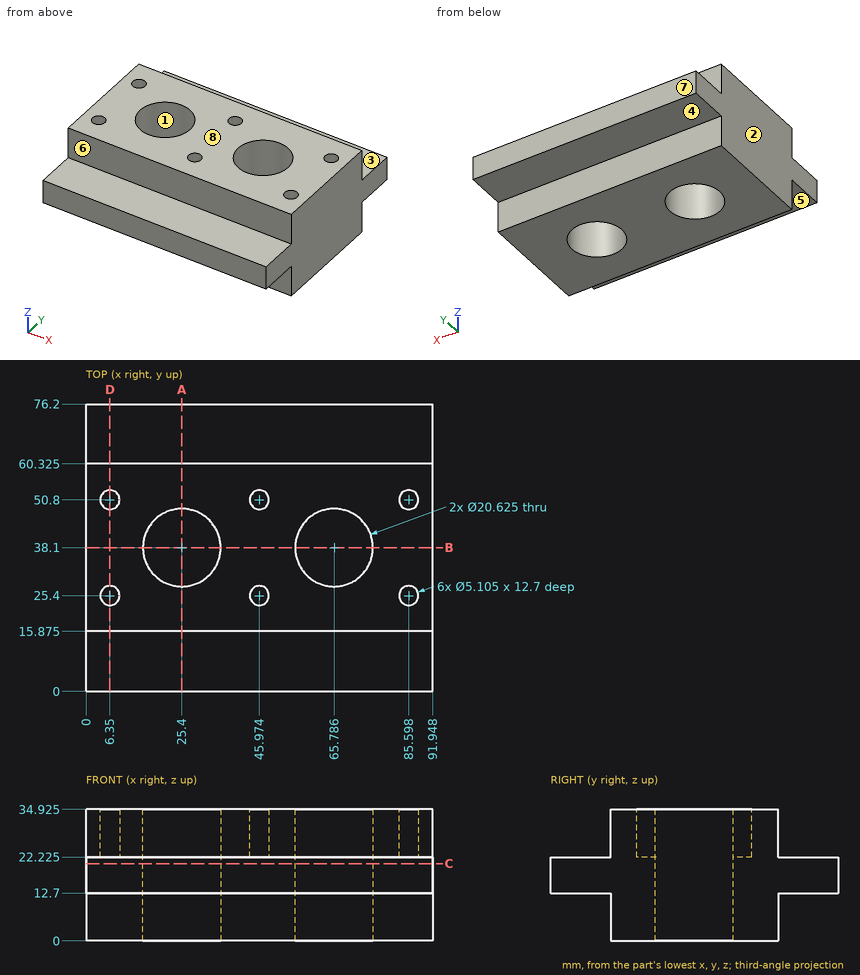
Input: dimensioned drawing with shaded views. Units: mm. Origin: part minimum x, y, z. A direction names the side the tool comes from. Give positions to 0.01 mm unless a question says otherwise; leave off trailing zeros. Order: outer loops, then holes, each group sorted by start corner. A loop starts at its lowest first (then second) coordinate and runs counter-clockwise, first axis right, second up. Notation, with made-up numbers: (-5.5, -9) -> (17.5, -9) arc R12 ccw to (17.5, 5) -> close; hole circle Ø6 at (68.5, 32.5). An arc over 180 degrees is marked (long way). Use a Markdown table: item, result.
1) Ray query, line 1 along X through (y, z) = (44, 12) (1 decimal); line 2 along X through (y, z) = (34, 24) (1 decimal); line 3 along Z through (x, y) = (24, 65.5) (1 decimal). Return the intervals inside material, ascending. Write a range as [from, to].
Answer list:
| item | result |
|---|---|
| line 1 | [0, 16.9], [33.9, 57.3], [74.2, 91.9] |
| line 2 | [0, 15.9], [34.9, 56.3], [75.2, 91.9] |
| line 3 | [12.7, 22.2] |
2) Section query D-D, the plane x = 6.35. Return the cut outline in (y, z) (1 decimal).
Answer list:
| item | result |
|---|---|
| outline | (0, 12.7) -> (15.9, 12.7) -> (15.9, 0) -> (60.3, 0) -> (60.3, 12.7) -> (76.2, 12.7) -> (76.2, 22.2) -> (60.3, 22.2) -> (60.3, 34.9) -> (53.4, 34.9) -> (53.4, 22.2) -> (48.2, 22.2) -> (48.2, 34.9) -> (28, 34.9) -> (28, 22.2) -> (22.8, 22.2) -> (22.8, 34.9) -> (15.9, 34.9) -> (15.9, 22.2) -> (0, 22.2) -> close |
3) Section query B-B, the plane y = 38.1. Return the cut outline in (x, z) (1 decimal).
Answer list:
| item | result |
|---|---|
| outline | (0, 0) -> (15.1, 0) -> (15.1, 34.9) -> (0, 34.9) -> close; (35.7, 0) -> (55.5, 0) -> (55.5, 34.9) -> (35.7, 34.9) -> close; (76.1, 0) -> (91.9, 0) -> (91.9, 34.9) -> (76.1, 34.9) -> close |
4) Section query C-C, the plane z = 20.5. Return the cut outline in (x, y) (1 decimal).
Answer list:
| item | result |
|---|---|
| outline | (0, 0) -> (91.9, 0) -> (91.9, 76.2) -> (0, 76.2) -> close; hole circle Ø20.6 at (25.4, 38.1); hole circle Ø20.6 at (65.8, 38.1) |
5) Reachability of the marked faces 4, 5, 6, 7 and 8 from +Z, -Z, +X, -X, +Y, -Y: full face, straight path, thin tool, end or side. Return the list, or none.
Answer list:
| item | result |
|---|---|
| face 4 | -Z, +X, -X, +Y |
| face 5 | -Z, +X, -X, -Y |
| face 6 | +Z, +X, -X, -Y |
| face 7 | +Z, -Z, +X, -X, +Y |
| face 8 | +Z, +X, -X, +Y, -Y |
6) Contact query for flat-ended pins moving along their axis: P1, Ø8, axis at x = 39.5, y = 6, coming from the +Z side (3 decimals); P2, Ø3, axis at x = 62.5, z = 6, coming from the +Y side (3 decimals); P3, Ø12.5, axis at x = 46.5, y = 68, coming from the -Z side. Output: stop coordinate, or through.
Answer list:
| item | result |
|---|---|
| P1 | z = 22.225 |
| P2 | y = 60.325 |
| P3 | z = 12.7 |
7) Section query A-A, the plane x = 25.4. Return the cut outline in (y, z) (1 decimal).
Answer list:
| item | result |
|---|---|
| outline | (0, 12.7) -> (15.9, 12.7) -> (15.9, 0) -> (27.8, 0) -> (27.8, 34.9) -> (15.9, 34.9) -> (15.9, 22.2) -> (0, 22.2) -> close; (48.4, 0) -> (60.3, 0) -> (60.3, 12.7) -> (76.2, 12.7) -> (76.2, 22.2) -> (60.3, 22.2) -> (60.3, 34.9) -> (48.4, 34.9) -> close |
8) Mould query, pull axis X, two halves, no side actions, for the marked faces 1, 2 and 3. Classes: +X half, -X half, draft (parallel to the pull), parting line (faces both ways), or undercut.
Answer list:
| item | result |
|---|---|
| face 1 | undercut |
| face 2 | -X half |
| face 3 | draft |
